Study the drawing (mm; zero at the part's minimum x, y, z) and answer. A direction names the side the tool comes from. Coordinates: 2 decimals unless noted, no trailing zeros. Write each loop counter-clockwise with the first axis right and the second up, starting at its lowest first coordinate (ties: lowest second). Pieces come first, ordered by that corner, then holes. Notation, with made-up numbers: (-27.75, 28.25) - (-10.75, 28.25) arc R23 cw to (-10.75, 54.25) - close; hole circle Ø3 at (-39, 44). An arc over 180 degrees is marked (long way). One line per item, written item: value.
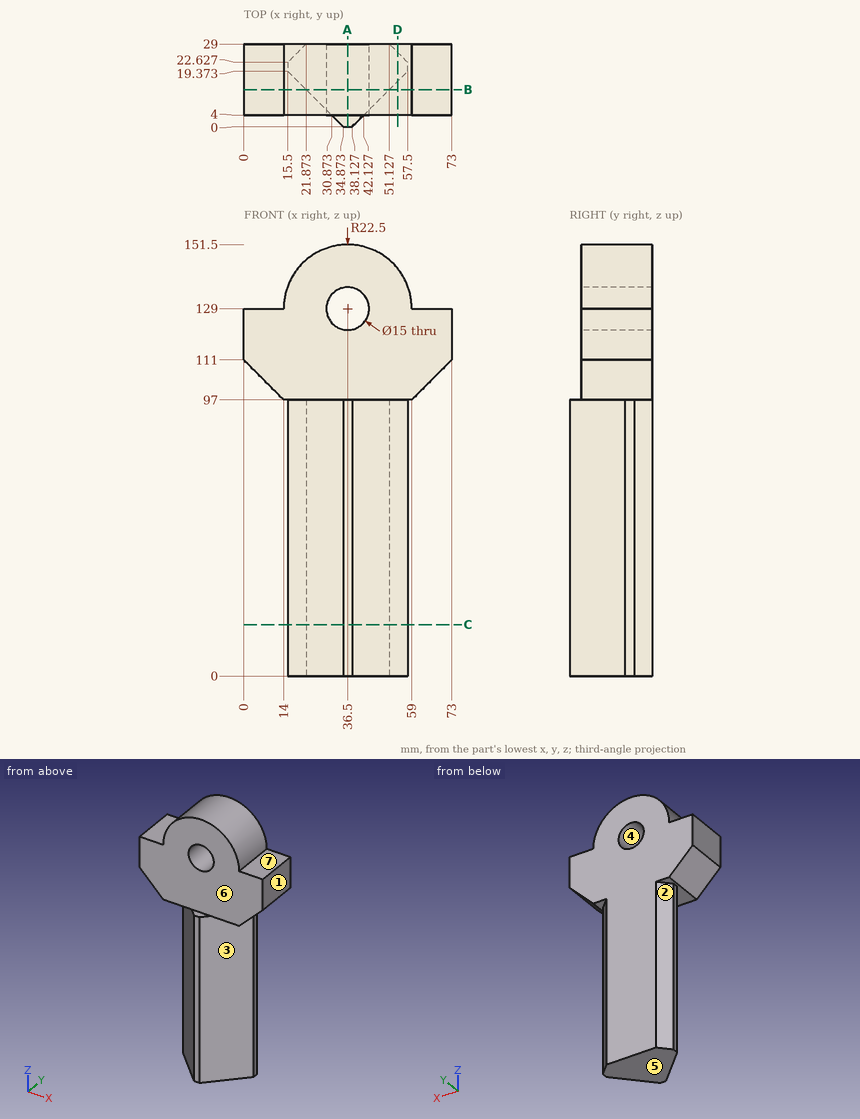
Item 1: Section B-B, the plane y = 13 is taken. Determine the outline of the cut face in (x, z), then the cut area to 3 significant figures.
Evaluation:
outline: (0, 111) - (14, 97) - (21.87, 97) - (21.87, 0) - (51.13, 0) - (51.13, 97) - (59, 97) - (73, 111) - (73, 129) - (59, 129) arc R22.5 ccw to (14, 129) - (0, 129) - close; hole circle Ø15 at (36.5, 129)
area: 5,600 mm2
Item 2: Section D-D, the plane x = 54 is taken. Determine the outline of the cut face in (y, z), then the cut area to 3 significant figures.
Evaluation:
outline: (4, 97) - (15.87, 97) - (15.87, 0) - (26.13, 0) - (26.13, 97) - (29, 97) - (29, 143.14) - (4, 143.14) - close
area: 2,150 mm2
Item 3: Consider probe 1 along Z at (x, y) = (36.5, 16.5); probe 2 along Y at (x, z) = (45, 100); probe 3 along Z at (x, y) = (34.5, 2.5). Determine where each line is inside the solid, lowest interval first.
Evaluation:
probe 1: z = 0 to 121.5, 136.5 to 151.5
probe 2: y = 4 to 29
probe 3: z = 0 to 97
Item 4: Section A-A, the plane x = 36.5 is taken. Determine the outline of the cut face in (y, z).
Evaluation:
outline: (0, 0) - (29, 0) - (29, 121.5) - (4, 121.5) - (4, 97) - (0, 97) - close; (4, 136.5) - (29, 136.5) - (29, 151.5) - (4, 151.5) - close
Item 5: Given pin 1 (3 mm diameter, centred on x = 33, y = 25, fed in from +Z); pin 2 (24 mm diameter, centred on x = 36.5, z = 129, fed in from -Y); pin 3 (4.5 mm diameter, centred on x = 35, y = 1.5, fed in from +Z), each flat-ended and moving along its own axis, determine where each tip first touches the part or whether it passes through.
Evaluation:
pin 1: stops at z = 151.41
pin 2: stops at y = 4
pin 3: stops at z = 97
Item 6: Which of the six approach directions +Z, -Z, +X, -X, +Y, -Y give full straight-line access (tool end or side, diameter ignored) to the marked faces 1, 2 and 3?
Evaluation:
face 1: +Z, -Z, +X, +Y, -Y
face 2: -Z, -X, +Y
face 3: -Z, +X, -Y
Item 7: Section C-C, the plane z = 18 is taken. Determine the outline of the cut face in (x, y), then the cut area to 3 significant figures.
Evaluation:
outline: (15.5, 19.37) - (34.87, 0) - (38.13, 0) - (57.5, 19.37) - (57.5, 22.63) - (51.13, 29) - (21.87, 29) - (15.5, 22.63) - close
area: 802 mm2
Item 8: Determine the mould class of the marked faces 4, 5, 6 and 7 for opening direction Z: +Z half, -Z half, draft (parallel to the pull), parting line (faces both ways), or undercut.
Evaluation:
face 4: undercut
face 5: -Z half
face 6: draft
face 7: +Z half
